```python
from build123d import *

# Parameters (mm, degrees)
SKETCH2_R               = 40
BOSS_EXTRUDE1_DEPTH     = 25
SKETCH3_R               = 47.5
BOSS_EXTRUDE2_DEPTH     = 2.5
CUT_EXTRUDE1_DEPTH      = 86.256964525
CUT_EXTRUDE1_DEPTH_BACK = 86.256964525
SKETCH4_W               = 30
SKETCH4_H               = 50


with BuildPart() as part:
    # Sketch2 → Boss-Extrude1 (new, symmetric)
    with BuildSketch(Plane(origin=(0, 0, 0), x_dir=(0, 0, -1), z_dir=(1, 0, 0))):
        Circle(SKETCH2_R)
    extrude(amount=BOSS_EXTRUDE1_DEPTH, both=True)

    # Sketch3 → Boss-Extrude2 (add, symmetric)
    with BuildSketch(Plane(origin=(25, 0, 0), x_dir=(0, 0, -1), z_dir=(1, 0, 0))):
        Circle(SKETCH3_R)
    boss_extrude2 = extrude(amount=BOSS_EXTRUDE2_DEPTH, both=True)

    # Mirror1: Boss-Extrude2 across plane
    add(boss_extrude2.mirror(Plane(origin=(0, 0, 0), x_dir=(0, 0, 1), z_dir=(1, 0, 0))))

    # Sketch4 → Cut-Extrude1 (cut, two sides: drawn at the far end of the back side and taken through both)
    with BuildSketch(Plane(origin=(25, 0, 0), x_dir=(0, 0, -1), z_dir=(1, 0, 0)).offset(-CUT_EXTRUDE1_DEPTH_BACK)):
        Rectangle(SKETCH4_W, SKETCH4_H)
    extrude(amount=CUT_EXTRUDE1_DEPTH + CUT_EXTRUDE1_DEPTH_BACK, mode=Mode.SUBTRACT)


solid = part.part
```
Geometry check sheet. Reference: the model listing, model coordinates, mm. A direction names the side the tool comes from. Round coordinates to 2 decimals unless told otherwise and drop trailing zeros. Write each loop counter-clockwise with the first axis right and the second up, starting at its lowest first coordinate (ties: lowest second). Pieces come first, ordered by that corner, then holes. Notation, with made-up numbers: (62, 39.25) -> (92, 39.25) arc R29 cw to (92, 61.25) -> close; hole circle Ø4 at (70, -7.75). An arc over 180 degrees is marked (long way). Put each result on its own line as item: value.
1) Cross-section at B-B, the plane z = 0. Enter the section's corners in (x, y).
Recorded:
outline: (-27.5, -47.5) -> (-22.5, -47.5) -> (-22.5, -40) -> (22.5, -40) -> (22.5, -47.5) -> (27.5, -47.5) -> (27.5, -25) -> (-27.5, -25) -> close; (-27.5, 25) -> (27.5, 25) -> (27.5, 47.5) -> (22.5, 47.5) -> (22.5, 40) -> (-22.5, 40) -> (-22.5, 47.5) -> (-27.5, 47.5) -> close
2) Release check for a two-part mould opening along X. For faces 1 (the face through (-27.5, 1, -20)), 2 (the face through (0, 0, 15)), 3 (the face through (-22.5, -35, 21)), 4 (the face through (22.5, -35, 21)) record: pulls with the +X half, pulls with the -X half, needs draft (parallel to the pull), parting line crosses it, or undercut.
Recorded:
face 1: pulls with the -X half
face 2: needs draft
face 3: undercut
face 4: undercut
3) Cross-section at C-C, the plane x = -15. Enter the section's corners in (y, z), plus the area to 3 significant figures.
Recorded:
outline: circle Ø80 at (0, 0); hole (-25, -15) -> (25, -15) -> (25, 15) -> (-25, 15) -> close
area: 3,530 mm2
4) Thickness scan on probe 1 along X at (y, z) = (19, -41.5); probe 2 along Y at (x, z) = (-3, -1); probe 3 along Z at (x, y) = (24, -18). Record the ranges inside material, lowest first. Write a range as from..to.
Recorded:
probe 1: x = -27.5..-22.5, 22.5..27.5
probe 2: y = -39.99..-25, 25..39.99
probe 3: z = -43.96..-15, 15..43.96
5) Depth check by flat-ended pin: P1, Ø15, axis at x = -9.5, z = -6, coming from the -Y side; P2, Ø1, axis at x = 21, y = 16, coming from the +Z side; P3, Ø10, axis at x = -20, y = -13.5, coming from the +Z side. Enter the tip coordinate at first touch or a pass-through.
Recorded:
P1: stops at y = -40
P2: stops at z = 36.87
P3: stops at z = 46.61
6) Access from +Z, -Z, +X, -X, +Y, -Y to the whole of each face (thin tool, end or side, straight path). Record for faces 5 (the face through (0, -25, 0)), 6 (the face through (27.5, 1, -20)), 7 (the face through (0.32, -39.05, 8.67)).
Recorded:
face 5: +X, -X
face 6: +Z, -Z, +X, +Y, -Y
face 7: none
7) Cross-section at A-A, the plane y = 0. Enter the section's corners in (x, z), plus the area to 3 significant figures.
Recorded:
outline: (-27.5, -47.5) -> (-22.5, -47.5) -> (-22.5, -40) -> (22.5, -40) -> (22.5, -47.5) -> (27.5, -47.5) -> (27.5, -15) -> (-27.5, -15) -> close; (-27.5, 15) -> (27.5, 15) -> (27.5, 47.5) -> (22.5, 47.5) -> (22.5, 40) -> (-22.5, 40) -> (-22.5, 47.5) -> (-27.5, 47.5) -> close
area: 2,900 mm2
8) Cross-section at D-D, the plane z = 25. Enter the section's corners in (x, y).
Recorded:
outline: (-27.5, -40.39) -> (-22.5, -40.39) -> (-22.5, -31.22) -> (22.5, -31.22) -> (22.5, -40.39) -> (27.5, -40.39) -> (27.5, 40.39) -> (22.5, 40.39) -> (22.5, 31.22) -> (-22.5, 31.22) -> (-22.5, 40.39) -> (-27.5, 40.39) -> close
